Drawing for the job (mm, zero at the part's lowest x, y, z). A direction names the side the tool comes from. Round coordinates to 2 decimals unless told otherwise and drop trailing zeros. Loops run counter-clockwise (first coordinate to the right, second up) from the corner with the lowest first, then second, coordinate; pieces in that order, holes last. Notation, with made-up numbers: M 65,-21 L 80,-21 A7 cw 80,-9 Z; hole C 73.25,54 d3. An arc over 180 degrees is marked long. Answer in a Markdown table with one row per item.
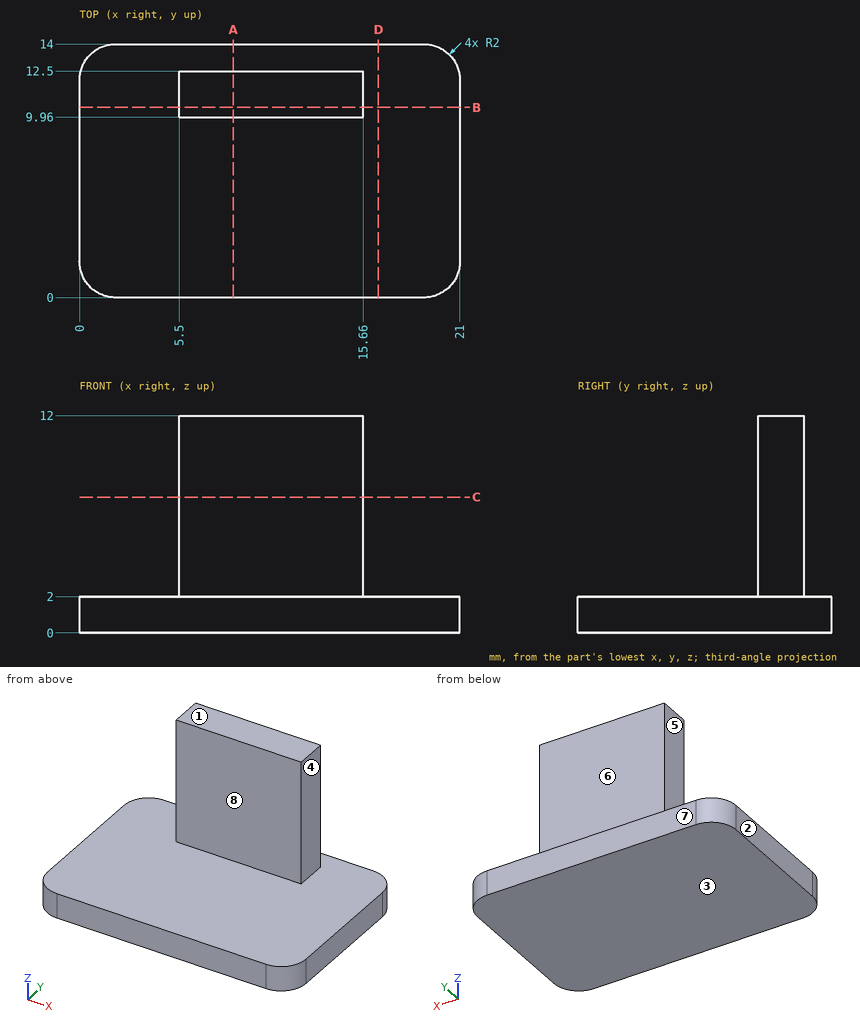
1. Saw through at B-B (y = 10.5). Write the cut outline in (x, z).
Verdict:
| item | result |
|---|---|
| outline | M 0,0 L 21,0 L 21,2 L 15.66,2 L 15.66,12 L 5.5,12 L 5.5,2 L 0,2 Z |
2. Wall check: probe 1 along Z at (x, y) = (9.5, 7.75); probe 2 along Y at (x, z) = (9.25, 10.75); probe 3 along X at (y, z) = (12.25, 2.75). Give the ranges that are in metal, low to high.
Verdict:
| item | result |
|---|---|
| probe 1 | z = 0 to 2 |
| probe 2 | y = 9.96 to 12.5 |
| probe 3 | x = 5.5 to 15.66 |
3. Tool access for the marked faces 4, 5, 6, 7 and 8: list every direction of +Z, -Z, +X, -X, +Y, -Y with a clear straight run to the whole face (end or side of a thin tool).
Verdict:
| item | result |
|---|---|
| face 4 | +Z, +X, +Y, -Y |
| face 5 | +Z, -X, +Y, -Y |
| face 6 | +Z, +X, -X, +Y |
| face 7 | +Z, -Z, +X, -X, +Y |
| face 8 | +Z, +X, -X, -Y |
4. Saw through at D-D (x = 16.5). Write the cut outline in (y, z), and give its area (3 significant figures).
Verdict:
| item | result |
|---|---|
| outline | M 0,0 L 14,0 L 14,2 L 0,2 Z |
| area | 28.0 mm² |
5. Saw through at A-A (x = 8.5). Write the cut outline in (y, z), and give its area (3 significant figures).
Verdict:
| item | result |
|---|---|
| outline | M 0,0 L 14,0 L 14,2 L 12.5,2 L 12.5,12 L 9.96,12 L 9.96,2 L 0,2 Z |
| area | 53.4 mm² |
6. Pin check, flat tips, straight feed: pin 1 (2 mm diameter, centred on y = 10.5, z = 9.5, fed in from -X); pin 2 (2 mm diameter, centred on x = 17, y = 3, fed in from +Z); pin 3 (3 mm diameter, centred on y = 2, z = 4.5, fed in from +X); pin 4 (2 mm diameter, centred on y = 11.5, z = 5, fed in from +X). Stop position of each tip, or through.
Verdict:
| item | result |
|---|---|
| pin 1 | stops at x = 5.5 |
| pin 2 | stops at z = 2 |
| pin 3 | passes through |
| pin 4 | stops at x = 15.66 |
7. Mould opens along Z. For the marked faces 1, 2 and 3 say: +Z half, -Z half, draft (parallel to the pull), parting line (faces both ways), or undercut.
Verdict:
| item | result |
|---|---|
| face 1 | +Z half |
| face 2 | draft |
| face 3 | -Z half |
8. Saw through at C-C (z = 7.5). Write the cut outline in (x, y).
Verdict:
| item | result |
|---|---|
| outline | M 5.5,9.96 L 15.66,9.96 L 15.66,12.5 L 5.5,12.5 Z |
